```python
from build123d import *

# Parameters (mm, degrees)
SKETCH1_R           = 10
BOSS_EXTRUDE1_DEPTH = 20
SKETCH2_R           = 3.125
CUT_EXTRUDE1_DEPTH  = 17
SKETCH3_R           = 6
CUT_EXTRUDE2_DEPTH  = 4


with BuildPart() as part:
    # Sketch1 → Boss-Extrude1 (new body)
    with BuildSketch(Plane(origin=(0, 0, 0), x_dir=(1, 0, 0), z_dir=(0, 1, 0))):
        with Locations(Location((0, 0, 0), (0, 0, 270))):  # turned: the seam where the file's is
            Circle(SKETCH1_R)
    extrude(amount=BOSS_EXTRUDE1_DEPTH)

    # Sketch2 → Cut-Extrude1 (cut)
    with BuildSketch(Plane.XZ):
        with Locations(Location((0, 0, 0), (0, 0, 270))):  # turned: the seam where the file's is
            Circle(SKETCH2_R)
    extrude(amount=-CUT_EXTRUDE1_DEPTH, mode=Mode.SUBTRACT)

    # Sketch3 → Cut-Extrude2 (cut)
    with BuildSketch(Plane.XZ):
        with Locations(Location((0, 0, 0), (0, 0, 270))):  # turned: the seam where the file's is
            Circle(SKETCH3_R)
    extrude(amount=-CUT_EXTRUDE2_DEPTH, mode=Mode.SUBTRACT)


solid = part.part
```
Could you check a few things on this model? Use its own coordinates, in mm. A direction names the side the tool comes from. Round coordinates to 2 decimals unless told otherwise and drop trailing zeros. Loops run counter-clockwise (first coordinate to the right, second up) from the corner with the lowest first, then second, coordinate; pieces in that order, holes last. Notation, with made-up numbers: (34.25, 50.5) -> (59.25, 50.5) arc R16 cw to (59.25, 62.5) -> close; hole circle Ø8 at (-3, -23). An arc over 180 degrees is marked (long way). One line per question, with ' | ' between items.
(1) If we section it at D-D on x = 4.75: List the corners of the cut face in (y, z) for me, and give its area (3 significant figures).
Model answer:
outline: (0, -8.8) -> (20, -8.8) -> (20, 8.8) -> (0, 8.8) -> (0, 3.67) -> (4, 3.67) -> (4, -3.67) -> (0, -3.67) -> close | area: 323 mm^2
(2) If I drill on probe 1 along X at (y, z) = (12, 0) (3 decimals); probe 2 along X at (y, z) = (2.85, 0); probe 3 along Y at (x, z) = (-1.75, 2), over which ranges is the centre line in solid material (lowest first)?
Model answer:
probe 1: x = -10 to -3.125, 3.125 to 10 | probe 2: x = -10 to -6, 6 to 10 | probe 3: y = 17 to 20
(3) If we section it at B-B on x = 0: List the corners of the cut face in (y, z) for me (3 decimals).
Model answer:
outline: (0, -10) -> (20, -10) -> (20, 10) -> (0, 10) -> (0, 6) -> (4, 6) -> (4, 3.125) -> (17, 3.125) -> (17, -3.125) -> (4, -3.125) -> (4, -6) -> (0, -6) -> close
(4) If we section it at C-C on y = 7.5: List the corners of the cut face in (x, z) for me (3 decimals).
Model answer:
outline: circle Ø20 at (0, 0); hole circle Ø6.25 at (0, 0)
(5) For pin 1 Ø6 at (x, z) = (-1, 0.5) entering from -Y; pin 2 Ø10 at (x, y) = (-7, 12) entering from +Z; pin 3 Ø9.5 at (x, z) = (-2, 3) entering from -Y; pin 4 Ø6 at (y, z) = (14.5, -4.5) entering from +X, each with a flat end and sliding along its axis, tell me the tip position at first contact or that it passes through.
Model answer:
pin 1: stops at y = 4 | pin 2: stops at z = 9.8 | pin 3: stops at y = 0 | pin 4: stops at x = 9.89
(6) If we section it at A-A on z = 0: List the corners of the cut face in (x, y) for me (3 decimals), and give its area (3 significant figures).
Model answer:
outline: (-10, 0) -> (-6, 0) -> (-6, 4) -> (-3.125, 4) -> (-3.125, 17) -> (3.125, 17) -> (3.125, 4) -> (6, 4) -> (6, 0) -> (10, 0) -> (10, 20) -> (-10, 20) -> close | area: 271 mm^2
(7) Thinking about a two-plate mould opening in X: for faces 1 (the face through (-9.76, 9.86, -2.17)), 2 (the face through (0, 20, 0)), 3 (the face through (0.94, 10.41, -2.98)), which applies, released by +X, released by -X, zero draft, split by the parting line, or undercut?
Model answer:
face 1: split by the parting line | face 2: zero draft | face 3: undercut
(8) For faces 4 (the face through (-3, 4, -3)), 5 (the face through (-7, 0, 0)), which set-ups out of +Z, -Z, +X, -X, +Y, -Y let a thin tool reach every point of the face, with its end or its side?
Model answer:
face 4: -Y | face 5: +Z, -Z, +X, -X, -Y
